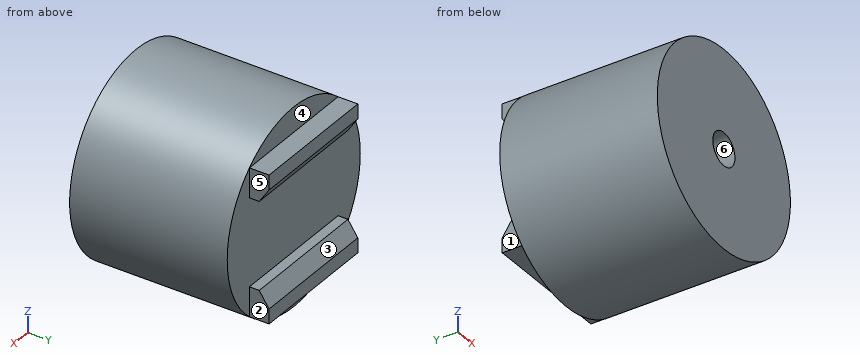
from build123d import *

# Parameters (mm, degrees)
SKETCH1_R           = 15
BOSS_EXTRUDE1_DEPTH = 24
SKETCH2_W           = 20
SKETCH2_H           = 4.5
BOSS_EXTRUDE2_DEPTH = 3
CUT_EXTRUDE1_DEPTH  = 43
SKETCH4_R           = 2.5
CUT_EXTRUDE2_DEPTH  = 7


with BuildPart() as part:
    # Sketch1 → Boss-Extrude1 (new body)
    with BuildSketch(Plane(origin=(0, 0, 0), x_dir=(1, 0, 0), z_dir=(0, 1, 0))):
        with Locations(Location((0, 0, 0), (0, 0, 270))):
            Circle(SKETCH1_R)
    extrude(amount=BOSS_EXTRUDE1_DEPTH)

    # Sketch2 → Boss-Extrude2 (add)
    with BuildSketch(Plane(origin=(0, 24, 0), x_dir=(1, 0, 0), z_dir=(0, 1, 0))):
        with Locations((0, 8.930339887)):
            Rectangle(SKETCH2_W, SKETCH2_H)
    extrude(amount=BOSS_EXTRUDE2_DEPTH)

    # Sketch3 → Cut-Extrude1 (cut)
    with BuildSketch(Plane(origin=(10, 0, 0), x_dir=(0, 0, -1), z_dir=(1, 0, 0))):
        Polygon((6.680339887, 25.5), (8.930339887, 27), (6.680339887, 27), align=None)
    extrude(amount=-CUT_EXTRUDE1_DEPTH, mode=Mode.SUBTRACT)

    # Mirror1: part across plane


with BuildPart() as part_1:
    add(part.part)
    add(part.part.mirror(Plane.XY))

    # Sketch4 → Cut-Extrude2 (cut)
    with BuildSketch(Plane.XZ):
        with Locations(Location((0, 0, 0), (0, 0, 270))):
            Circle(SKETCH4_R)
    extrude(amount=-CUT_EXTRUDE2_DEPTH, mode=Mode.SUBTRACT)


solid = part_1.part
Could you check a few things on this model? Use its own coordinates, in mm. Face numbers are marked on the shaded views. A direction names the side the tool comes from. Round coordinates to 2 decimals unless told otherwise and drop trailing zeros. Order: outer loops, then holes, each group sorted by start corner. A loop starts at its lowest first (then second) coordinate and runs counter-clockwise, first axis right, second up.
Q1. Which directions (+Z, -Z, +X, -X, +Y, -Y) give clear straight access to the entire face, cutting with the end or side of a thin tool? Please do the marked faces 1, 2 and 3.
Geometry says:
face 1: +Z, -Z, -X, +Y
face 2: +Z, -Z, +X, +Y
face 3: +X, -X, +Y
Q2. Imagine slicing it at D-D, the plane x = 0. List the corners of the cut face in (y, z) for me, then the cut area to 3 significant figures.
Geometry says:
outline: (0, -15) - (24, -15) - (24, -11.18) - (27, -11.18) - (27, -8.93) - (25.5, -6.68) - (24, -6.68) - (24, 6.68) - (25.5, 6.68) - (27, 8.93) - (27, 11.18) - (24, 11.18) - (24, 15) - (0, 15) - (0, 2.5) - (7, 2.5) - (7, -2.5) - (0, -2.5) - close
area: 709 mm2
Q3. Imagine slicing it at C-C, the plane y = 17. List the corners of the cut face in (x, z) for me, then the cut area to 3 significant figures.
Geometry says:
outline: circle Ø30 at (0, 0)
area: 707 mm2
Q4. I'm going to push flat-ended pins straight in: P1, Ø6.5, axis at x = 5.5, z = -0.5, coming from the +Y side; P2, Ø0.9, axis at y = 25, z = 8, coming from the -X side; P3, Ø3.5, axis at x = 2, y = 26, coming from the +Z side. Where does each tip first touch, or does it pass through?
Geometry says:
P1: stops at y = 24
P2: stops at x = -10
P3: stops at z = 11.18
Q5. Please list where these lines run through material, in increasing order: probe 1 along X at (y, z) = (5, 0); probe 2 along Z at (x, y) = (2.5, 24.25); probe 3 along Y at (x, z) = (-9.5, 4.75).
Geometry says:
probe 1: x = -15 to -2.5, 2.5 to 15
probe 2: z = -11.18 to -6.68, 6.68 to 11.18
probe 3: y = 0 to 24
Q6. Imagine slicing it at A-A, the plane x = 9. List the corners of the cut face in (y, z) for me.
Geometry says:
outline: (0, -12) - (24, -12) - (24, -11.18) - (27, -11.18) - (27, -8.93) - (25.5, -6.68) - (24, -6.68) - (24, 6.68) - (25.5, 6.68) - (27, 8.93) - (27, 11.18) - (24, 11.18) - (24, 12) - (0, 12) - close
Q7. Imagine slicing it at B-B, the plane z = 0. List the corners of the cut face in (x, y) for me, then the cut area to 3 significant figures.
Geometry says:
outline: (-15, 0) - (-2.5, 0) - (-2.5, 7) - (2.5, 7) - (2.5, 0) - (15, 0) - (15, 24) - (-15, 24) - close
area: 685 mm2
Q8. Thinking about a two-plate mould opening in X: for the marked faces 4, 5 and 6, which applies, released by +X, released by -X, zero draft, split by the parting line, or undercut?
Geometry says:
face 4: zero draft
face 5: released by +X
face 6: undercut
